Part model, mm, in its own coordinate system. A direction names the side the tool comes from. Give positions to 0.01 mm unless a question says otherwise; leave off trailing zeros. Write each loop counter-clockwise with the first axis right and the second up, starting at its lowest first coordinate (ties: lowest second). Pieces come first, ordered by that corner, then holes.
from build123d import *

# Parameters (mm, degrees)
F0_W     = 7
F0_H     = 6
F2_DEPTH = 7
F1_W     = 7
F1_H     = 7
F3_DEPTH = 10


with BuildPart() as f2:
    # F0 (on Front) → F2 (new body)
    with BuildSketch(Plane.XZ):
        Rectangle(F0_W, F0_H)
    extrude(amount=F2_DEPTH)

    # F1 (on Front) → F3 (join)
    with BuildSketch(Plane.XZ):
        with Locations((0, -6.045629)):
            Rectangle(F1_W, F1_H)
    extrude(amount=F3_DEPTH)


solid = f2.part
1) Flat gauge pins, fed straight in: P1, Ø2.5, axis at x = 1, y = -9, coming from the +Z side; P2, Ø1.7, axis at x = 0.5, z = 0, coming from the -Y side. Where does each tip first touch, or does it go through?
Check result:
P1: stops at z = -2.55
P2: stops at y = -7
2) Saw through at A-A (y = -7.25). Write the cut outline in (x, z).
Check result:
outline: (-3.5, -9.55) - (3.5, -9.55) - (3.5, -2.55) - (-3.5, -2.55) - close
3) Drill centre lines: L1, parallel to Z at x = -1, y = -8.25; L2, parallel to Y at x = 1.75, z = -0.75. Where is each one in solid material? Low to high.
Check result:
L1: z = -9.55 to -2.55
L2: y = -7 to 0
4) 3-axis set-ups, long thin cutter, end or side, ignore diameter. For faces 1 (the flat face through (0, 0, -3)), 2 (the flat face through (0, -7, 0)): which of +Z, -Z, +X, -X, +Y, -Y reach the whole face in a straight line?
Check result:
face 1: +Z, -Z, +X, -X, +Y
face 2: +Z, +X, -X, -Y
5) Saw through at B-B (x = 0.5). Write the cut outline in (y, z).
Check result:
outline: (-10, -9.55) - (0, -9.55) - (0, 3) - (-7, 3) - (-7, -2.55) - (-10, -2.55) - close
6) Saw through at C-C (z = -0.25). Write the cut outline in (x, y), and give its area (3 significant figures).
Check result:
outline: (-3.5, -7) - (3.5, -7) - (3.5, 0) - (-3.5, 0) - close
area: 49.0 mm2
